from build123d import *

# Parameters (mm, degrees)
F0_W     = 19.07
F0_H     = 10.5
F1_DEPTH = 10.5
F2_R     = 3.525
F3_DEPTH = 10.5
F4_R     = 3.525
F5_DEPTH = 9
F7_DEPTH = 10.501


with BuildPart() as f1:
    # F0 (on Front) → F1 (new body)
    with BuildSketch(Plane.XZ):
        Rectangle(F0_W, F0_H)
    extrude(amount=-F1_DEPTH)

    # F2 (on face) → F3 (cut, through all)
    with BuildSketch(Plane.XZ):
        with BuildLine():
            ThreePointArc((-4.285, -5.25), (-7.997311, -3.712311), (-9.535, 0))
            Line((-9.535, 0), (-9.535, -5.25))
            Line((-9.535, -5.25), (-4.285, -5.25))
        make_face()
        with BuildLine():
            ThreePointArc((-9.535, 0), (-7.997311, 3.712311), (-4.285, 5.25))
            Line((-4.285, 5.25), (-9.535, 5.25))
            Line((-9.535, 5.25), (-9.535, 0))
        make_face()
        with Locations((-4.285, 0)):
            Circle(F2_R)
    extrude(amount=-F3_DEPTH, mode=Mode.SUBTRACT)

    # F4 (on face) → F5 (cut)
    with BuildSketch(Plane.XY.offset(5.25)):
        with Locations((4.285, 5.25)):
            Circle(F4_R)
    extrude(amount=-F5_DEPTH, mode=Mode.SUBTRACT)

    # F6 (on face) → F7 (cut, through all)
    with BuildSketch(Plane.XY.offset(5.25)):
        with BuildLine():
            ThreePointArc((4.285, 10.5), (7.997311, 8.962311), (9.535, 5.25))
            Line((9.535, 5.25), (9.535, 10.5))
            Line((9.535, 10.5), (4.285, 10.5))
        make_face()
        with BuildLine():
            ThreePointArc((9.535, 5.25), (7.997311, 1.537689), (4.285, 0))
            Line((4.285, 0), (9.535, 0))
            Line((9.535, 0), (9.535, 5.25))
        make_face()
    extrude(amount=-F7_DEPTH, mode=Mode.SUBTRACT)


solid = f1.part
Input: part model. Units: mm. Frame: model coordinates. A direction names the side the tool comes from. Round coordinates to 2 decimals unless told otherwise and drop trailing zeros. Write each loop counter-clockwise with the first axis right and the second up, starting at its lowest first coordinate (ties: lowest second). Pieces come first, ordered by that corner, then holes.
1) Reachability of faces 3 (the flat face through (4, 5, -3.75)), 4 (the flat face through (0, 10.5, 0)) from +Z, -Z, +X, -X, +Y, -Y: full face, straight path, thin tool, end or side. Return the list, or none.
2) Contact query for flat-ended pins moving along their axis: P1, Ø1.5, axis at y = 4, z = -1, coming from the -X side; P2, Ø2, axis at x = 3.5, y = 5.5, coming from the +Z side. Output: stop coordinate, or through.
3) Ray query, L1, parallel to X at y = 4, z = -2.5; L2, parallel to X at y = 2.75, z = 2.5; L3, parallel to Y at x = 5.5, z = -1.25. Return the intervals inside material, ascending.
4) Cut plane D-D (x = 4). Return the cut outline in (y, z).
5) Cut plane A-A (z = 0.75). Return the cut outline in (x, y) (3 decimals), then the cut area to 3 significant figures.
6) Cut plane C-C (y = 8). Return the cut outline in (x, z) (3 decimals).
7) Draft query along X for faces 1 (the cylindrical face through (3.52, 1.81, 0.81)), 2 (the flat face through (3, 5, -5.25)). Return one class per face: pulls with the +X half, pulls with the -X half, needs draft (parallel to the pull), parting line crosses it, or undercut.
8) Cut plane B-B (x = -3.25). Return the cut outline in (y, z).
Geometry says:
1. face 3: +Z
1. face 4: +Z, -Z, +X, -X, +Y
2. P1: stops at x = -9.53
2. P2: stops at z = -3.75
3. L1: x = -8.9 to -6.77, -1.8 to 0.99, 7.58 to 9.38
3. L2: x = -8.9 to -6.77, -1.8 to 1.8, 6.77 to 8.9
3. L3: y = 0.14 to 1.94, 8.56 to 10.36
4. outline: (0, -5.25) - (10.5, -5.25) - (10.5, 5.25) - (8.76, 5.25) - (8.76, -3.75) - (1.74, -3.75) - (1.74, 5.25) - (0, 5.25) - close
5. outline: (-9.481, 0) - (-7.729, 0) - (-7.729, 10.5) - (-9.481, 10.5) - close; (-0.841, 0) - (4.285, 0) arc R5.25 ccw to (9.535, 5.25) arc R5.25 ccw to (4.285, 10.5) - (-0.841, 10.5) - close; hole circle Ø7.05 at (4.285, 5.25)
5. area: 76.5 mm2
6. outline: (-9.535, 0) arc R5.25 ccw to (-4.285, -5.25) - (8.757, -5.25) - (8.757, 5.25) - (6.49, 5.25) - (6.49, -3.75) - (2.08, -3.75) - (2.08, 5.25) - (-4.285, 5.25) arc R5.25 ccw to start; hole circle Ø7.05 at (-4.285, 0)
7. face 1: undercut
7. face 2: needs draft
8. outline: (0, -5.25) - (10.5, -5.25) - (10.5, -3.37) - (0, -3.37) - close; (0, 3.37) - (10.5, 3.37) - (10.5, 5.25) - (0, 5.25) - close
